from build123d import *

# Parameters (mm, degrees)
SKETCH1_W             = 100
SKETCH1_H             = 75
PLATE_DEPTH           = 6.35
SKETCH2_R             = 2.5
CUT_IDLER_HOLES_DEPTH = 126.161186076
SKETCH3_R             = 1.5
SKETCH3_R_2           = 11.5
CUT_MOTOR_HOLES_DEPTH = 126.161186076
CHAMFER1_SIZE         = 1.5
FILLET1_R             = 10
CUT_EXTRUDE1_DEPTH    = 6.35
FILLET5_R             = 10


with BuildPart() as part:
    # Sketch1 → plate (new body)
    with BuildSketch(Plane.XY):
        with Locations((50, 37.5)):
            Rectangle(SKETCH1_W, SKETCH1_H)
    extrude(amount=PLATE_DEPTH)

    # Sketch2 → cut idler holes (cut, through all)
    with BuildSketch(Plane.XY.offset(6.35)):
        with Locations((54, 62.5)):
            Circle(SKETCH2_R)
        with Locations((12, 37.5)):
            Circle(SKETCH2_R)
        with Locations((54, 12.5)):
            Circle(SKETCH2_R)
    extrude(amount=-CUT_IDLER_HOLES_DEPTH, mode=Mode.SUBTRACT)

    # Sketch3 → cut motor holes (cut, through all)
    with BuildSketch(Plane.XY.offset(6.35)):
        with Locations((57.5, 53)):
            Circle(SKETCH3_R)
        with Locations((88.5, 53)):
            Circle(SKETCH3_R)
        with Locations((88.5, 22)):
            Circle(SKETCH3_R)
        with Locations((57.5, 22)):
            Circle(SKETCH3_R)
        with Locations((73, 37.5)):
            Circle(SKETCH3_R_2)
    extrude(amount=-CUT_MOTOR_HOLES_DEPTH, mode=Mode.SUBTRACT)

    # Chamfer1
    chamfer1_edges = [part.edges().sort_by_distance(p)[0] for p in [
        (56, 53, 0),
        (87, 22, 0),
        (56, 22, 0),
        (87, 53, 0),
    ]]
    chamfer(chamfer1_edges, length=CHAMFER1_SIZE)

    # Fillet1
    fillet1_edges = [part.edges().sort_by_distance(p)[0] for p in [
        (0, 75, 3.175),
        (100, 75, 3.175),
        (100, 0, 3.175),
        (0, 0, 3.175),
    ]]
    fillet(fillet1_edges, radius=FILLET1_R)

    # Sketch4 → Cut-Extrude1 (cut)
    with BuildSketch(Plane.XY.offset(6.35)):
        with BuildLine():
            Line((10, 0), (21, 0))
            Line((21, 0), (0, 37.5))
            Line((0, 37.5), (0, 10))
            ThreePointArc((0, 10), (2.928932188, 2.928932188), (10, 0))
        make_face()
    cut_extrude1 = extrude(amount=-CUT_EXTRUDE1_DEPTH, mode=Mode.SUBTRACT)

    # Mirror2: Cut-Extrude1 across plane
    add(cut_extrude1.mirror(Plane(origin=(0, 37.5, 0), x_dir=(0, 0, 1), z_dir=(0, -1, 0))), mode=Mode.SUBTRACT)

    # Fillet5
    fillet5_edges = [part.edges().sort_by_distance(p)[0] for p in [
        (21, 75, 3.175),
        (0, 37.5, 3.175),
        (21, 0, 3.175),
    ]]
    fillet(fillet5_edges, radius=FILLET5_R)


solid = part.part
For this review, take the finished solid that the model builds, in its own axes (mm). Give positions to 0.01 mm unless a question says otherwise; leave off trailing zeros. Loops run counter-clockwise (first coordinate to the right, second up) from the corner with the lowest first, then second, coordinate; pieces in that order, holes last.
Item 1: Insertion check: pin 1 (2 mm diameter, centred on y = 16.5, z = 1.5, fed in from -X); pin 2 (4 mm diameter, centred on x = 57.5, y = 22, fed in from -Z); pin 3 (1 mm diameter, centred on x = 17.5, z = 2.5, fed in from -Y). Each pin has a flat end and moves straight along its axis. Give the tip position at first contact, or say it passes through.
Item 2: For line 1 along Y through (x, z) = (57.5, 4.05); line 2 along Y through (x, z) = (73.5, 5.5); line 3 along X through (y, z) = (46, 2.25), list the stretches that pass through material, from the lowest coordinate up.
Item 3: Take a section at D-D, the plane x = 70. State the section outline as (y, z) points.
Item 4: Take a section at B-B, the plane z = 3.25. Give the number of separate pieces and of enclosed holes in the cut face, and give its area (3 significant figures).
Item 5: Draft analysis for pull direction X (two halves, no side actions). For faces 1 (the cylindrical face through (1.46, 37.57, 3.13)), 2 (the flat face through (100, 37, 3)), 3 (the cylindrical face through (63.874, 30.502, 3.219)), 4 (the flat face through (50, 38, 6.35)), state which applies: +X half, -X half, draft (parallel to the pull), parting line (faces both ways), or undercut.
Item 6: Take a section at A-A, the plane y = 22. State the section outline as (x, z) points.
Item 7: Take a section at C-C, the plane y = 12.5. State the section outline as (x, z) points.
Calculated:
1. pin 1: stops at x = 11.2
1. pin 2: stops at z = 1
1. pin 3: stops at y = 5.36
2. line 1: y = 0 to 20.5, 23.5 to 51.5, 54.5 to 75
2. line 2: y = 0 to 26.01, 48.99 to 75
2. line 3: x = 4.76 to 65.25, 80.75 to 100
3. outline: (0, 0) - (26.4, 0) - (26.4, 6.35) - (0, 6.35) - close; (48.6, 0) - (75, 0) - (75, 6.35) - (48.6, 6.35) - close
4. separate pieces: 1
4. enclosed holes: 8
4. area: 6,150 mm2
5. face 1: -X half
5. face 2: +X half
5. face 3: undercut
5. face 4: draft
6. outline: (8.68, 0) - (54.5, 0) - (56, 1.5) - (56, 6.35) - (8.68, 6.35) - close; (59, 1.5) - (60.5, 0) - (85.5, 0) - (87, 1.5) - (87, 6.35) - (59, 6.35) - close; (90, 1.5) - (91.5, 0) - (100, 0) - (100, 6.35) - (90, 6.35) - close
7. outline: (14, 0) - (51.5, 0) - (51.5, 6.35) - (14, 6.35) - close; (56.5, 0) - (100, 0) - (100, 6.35) - (56.5, 6.35) - close
